from build123d import *

# Parameters (mm, degrees)
SKETCH1_W                    = 390
SKETCH1_H                    = 90
BOSS_EXTRUDE1_DEPTH          = 3.175
CSK_FOR_M4_SFHCS1_AT_2_COUNT = 2
CSK_FOR_M4_SFHCS1_AT_2_PITCH = 388.329756779
CSK_FOR_M4_SFHCS1_AT_3_COUNT = 2
CSK_FOR_M4_SFHCS1_AT_3_PITCH = 380
CSK_FOR_M4_SFHCS1_AT_4_COUNT = 2
CSK_FOR_M4_SFHCS1_AT_4_PITCH = 80


with BuildPart() as part:
    # Sketch1 → Boss-Extrude1 (new body)
    with BuildSketch(Plane.XY):
        Rectangle(SKETCH1_W, SKETCH1_H)
    extrude(amount=BOSS_EXTRUDE1_DEPTH)

    # Sketch3 → CSK for M4 SFHCS1 (revolve, cut)
    with BuildSketch(Plane(origin=(190, 40, 3.175), x_dir=(0, -1, 0), z_dir=(1, 0, 0))):
        Polygon((0, 0), (0, 3.175), (2.25, 3.175), (2.25, 2.23), (4.48, 0), align=None)
    csk_for_m4_sfhcs1 = revolve(axis=Axis((190, 40, 9.525), (0, 0, -1)), mode=Mode.SUBTRACT)

    # CSK for M4 SFHCS1 at 2: CSK for M4 SFHCS1 ×2
    with Locations(*[Vector(-0.9785497849867489, -0.20601048104984204, 0) * (i * CSK_FOR_M4_SFHCS1_AT_2_PITCH) for i in range(1, CSK_FOR_M4_SFHCS1_AT_2_COUNT)]):
        add(csk_for_m4_sfhcs1, mode=Mode.SUBTRACT)

    # CSK for M4 SFHCS1 at 3: CSK for M4 SFHCS1 ×2
    with Locations(*[(-i * CSK_FOR_M4_SFHCS1_AT_3_PITCH, 0, 0) for i in range(1, CSK_FOR_M4_SFHCS1_AT_3_COUNT)]):
        add(csk_for_m4_sfhcs1, mode=Mode.SUBTRACT)

    # CSK for M4 SFHCS1 at 4: CSK for M4 SFHCS1 ×2
    with Locations(*[(0, -i * CSK_FOR_M4_SFHCS1_AT_4_PITCH, 0) for i in range(1, CSK_FOR_M4_SFHCS1_AT_4_COUNT)]):
        add(csk_for_m4_sfhcs1, mode=Mode.SUBTRACT)


solid = part.part
Verification items for the finished model (mm, model axes). Coordinates: 2 decimals unless noted, no trailing zeros. One line per item, written item: value. Start each with the question number.
Item 1: Scan lines: probe 1 along Y at (x, z) = (-190, 0.2); probe 2 along X at (y, z) = (-40, 0.5); probe 3 along X at (y, z) = (-41, 1.95). Record each from-to range of solid material in increasing order.
Item 2: Mould release check, pull along Y, two halves, no side actions. Record for faces 1 (the flat face through (-3, 1, 0)), 2 (the conical face through (192.33, -39.48, 1.08)): released by +Y, released by -Y, zero draft, split by the parting line, or undercut.
Item 3: Gauge pin test, flat end, axial feed: pin 1 (6 mm diameter, centred on x = 190, y = 40, fed in from +Z) (3 decimals). Record the tip position at first contact, or that the pin passes through.
Conclusion:
1. probe 1: y = -45 to -42.25, -37.75 to 37.75, 42.25 to 45
1. probe 2: x = -195 to -192.25, -187.75 to 187.75, 192.25 to 195
1. probe 3: x = -195 to -193.1, -186.9 to 186.9, 193.1 to 195
2. face 1: zero draft
2. face 2: undercut
3. pin 1: stops at z = 1.695
